Part model, mm, in its own coordinate system. Give positions to 0.01 mm unless a question says otherwise; leave off trailing zeros. Order: outer loops, then holes, each group sorted by start corner. A loop starts at its lowest first (then second) coordinate and runs counter-clockwise, first axis right, second up. Notation, with made-up numbers: M 23,30.5 L 81,30.5 A31 cw 81,64.5 Z; hole C 35,35 d10. An arc over 180 degrees is marked long. One line per question, with ' | ' between items.
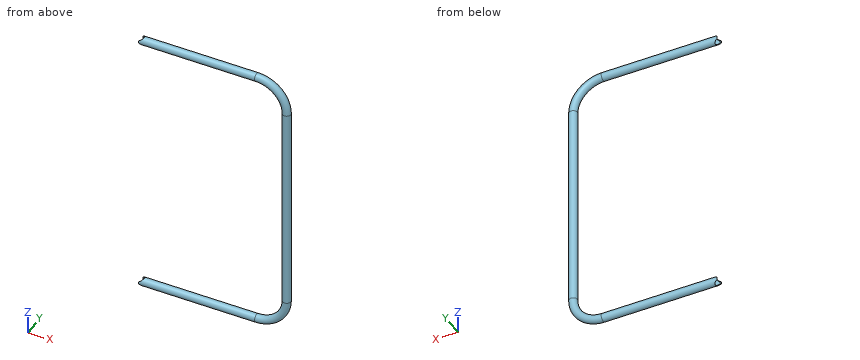
```python
from build123d import *

# Parameters (mm, degrees)
SKETCH_1_R    = 13.5
SKETCH_1_R_2  = 12
OTHER_START   = -9e-09
OTHER_1_DEPTH = 27.000000009


# Read off the part's stored shape, not the designer's step: Полость1
with BuildPart() as part:
    # По траектории1: sweep along a path in Эскиз2
    with BuildLine(Plane(origin=(0, 0, 0), x_dir=(1, 0, 0), z_dir=(0, 1, 0))) as sweep_1_path:
        Line((0, -13.5), (385.446701658, -13.5))
        ThreePointArc((385.446701658, -13.5), (456.157379776, 15.789321881), (485.446701658, 86.5))
        Line((485.446701658, 86.5), (485.446701658, 435))
    # Эскиз1 → По траектории1 (sweep)
    with BuildSketch(Plane(origin=(0, 0, 0), x_dir=(0, 0, -1), z_dir=(1, 0, 0))):
        with Locations((-13.5, 0)):
            Circle(SKETCH_1_R)
        with Locations((-13.5, 0)):
            Circle(SKETCH_1_R_2, mode=Mode.SUBTRACT)
    sweep(path=sweep_1_path.line)

    # Полость1 outline → Полость1 (cut)
    with BuildSketch(Plane.XY.offset(OTHER_START)):
        with BuildLine():
            Line((0, 12.5), (0, -12.5))
            ThreePointArc((0, -12.5), (12.5, 0), (0, 12.5))
        make_face()
    extrude(amount=OTHER_1_DEPTH, mode=Mode.SUBTRACT)

    # Зеркальное отражение1: part across plane


with BuildPart() as part_1:
    add(part.part)
    add(part.part.mirror(Plane(origin=(485.446701658, 0, -435), x_dir=(1, 0, 0), z_dir=(0, 0, -1))))


solid = part_1.part
```
1. Slice it at C-C on z = -464.5. Give the cut face in (x, y).
Worked out:
outline: C 485.45,0 d27; hole C 485.45,0 d24
2. Slice it at B-B on y = 0. Give the cut face in (x, z).
Worked out:
outline: M 12.5,-897 L 385.45,-897 A113.5 ccw 498.95,-783.5 L 498.95,-86.5 A113.5 ccw 385.45,27 L 12.5,27 L 12.5,25.5 L 385.45,25.5 A112 cw 497.45,-86.5 L 497.45,-783.5 A112 cw 385.45,-895.5 L 12.5,-895.5 Z; M 12.5,-871.5 L 385.45,-871.5 A88 ccw 473.45,-783.5 L 473.45,-86.5 A88 ccw 385.45,1.5 L 12.5,1.5 L 12.5,0 L 385.45,0 A86.5 cw 471.95,-86.5 L 471.95,-783.5 A86.5 cw 385.45,-870 L 12.5,-870 Z
3. Slice it at A-A on x = 302. Give the cut face in (y, z), then the cut area to 3 significant figures.
Worked out:
outline: C 0,-883.5 d27; C 0,13.5 d27; hole C 0,-883.5 d24; hole C 0,13.5 d24 | area: 240 mm2
4. Drop flat-ended pins along their axis: pin 1 (3 mm diameter, centred on x = 64.5, y = 9, fed in from -Z) (3 decimals); pin 2 (4 mm diameter, centred on x = 148, y = 5, fed in from +Z); pin 3 (6 mm diameter, centred on x = 258.5, y = 1, fed in from -Z); pin 4 (1 mm diameter, centred on y = 9, z = -526, fed in from +X). Give the stop position or say it passes through.
Worked out:
pin 1: stops at z = -894.725 | pin 2: stops at z = 26.66 | pin 3: stops at z = -897 | pin 4: stops at x = 495.93
5. Probe L1, parallel to Z at x = 85, y = 0.75; L2, parallel to Z at x = 271, y = -1.5; L3, parallel to X at y = -2, z = -651.5. List the from-to ranges inside material, lowest first. Write a range as from..to.
Worked out:
L1: z = -896.98..-895.48, -871.52..-870.02, 0.02..1.52, 25.48..26.98 | L2: z = -896.92..-895.41, -871.59..-870.08, 0.08..1.59, 25.41..26.92 | L3: x = 472.1..473.61, 497.28..498.8
